The model under review builds one solid part; all positions refer to its coordinate system, in mm. Face numbers are marked on the shaded views. A direction names the side the tool comes from. Round coordinates to 2 decimals unless told otherwise and drop trailing zeros. Order: outer loops, then holes, each group sorted by start corner. A loop starts at its lowest first (then second) coordinate and runs counter-clockwise, first axis right, second up.
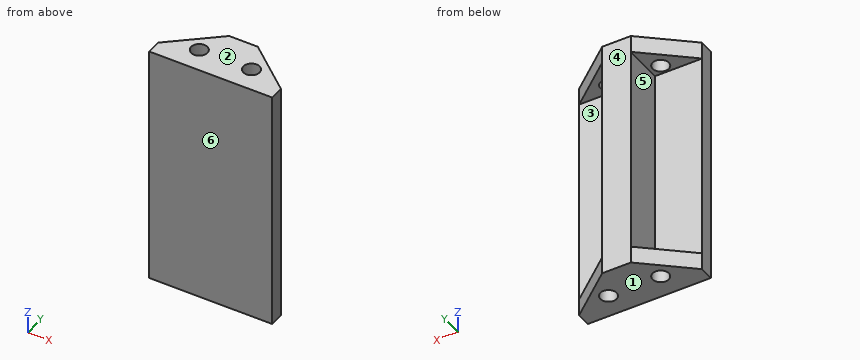
from build123d import *

# Parameters (mm, degrees)
SKETCH1_R           = 2.85
BOSS_EXTRUDE1_DEPTH = 85.7063165
CUT_EXTRUDE1_START  = -6
CUT_EXTRUDE1_DEPTH  = 73.706316
SKETCH3_R           = 2.85
CUT_EXTRUDE2_DEPTH  = 86.7063165


with BuildPart() as part:
    # Sketch1 → Boss-Extrude1 (new body)
    with BuildSketch(Plane.XY):
        Polygon((-21.5, -9.422571957), (21.5, -9.422571957), (21.5, -4.422571957), (5, 9.422571957), (-5, 9.422571957), (-21.5, -4.422571957), align=None)
        with Locations((-9.125, -0.961285979)):
            Circle(SKETCH1_R, mode=Mode.SUBTRACT)
        with Locations((9.125, -0.961285979)):
            Circle(SKETCH1_R, mode=Mode.SUBTRACT)
        with Locations((-9.125, -0.961285979)):
            Circle(SKETCH1_R)
        with Locations((9.125, -0.961285979)):
            Circle(SKETCH1_R)
    extrude(amount=BOSS_EXTRUDE1_DEPTH)

    # Sketch2 → Cut-Extrude1 (cut)
    with BuildSketch(Plane(origin=(0, 0, 0), x_dir=(-1, 0, 0), z_dir=(0, 0, -1)).offset(CUT_EXTRUDE1_START)):
        Polygon((5, 9.422571957), (21.5, -4.422571957), (5, -4.422571957), align=None)
        Polygon((-21.5, -4.422571957), (-5, 9.422571957), (-5, -4.422571957), align=None)
    extrude(amount=-CUT_EXTRUDE1_DEPTH, mode=Mode.SUBTRACT)

    # Sketch3 → Cut-Extrude2 (cut, through all)
    with BuildSketch(Plane(origin=(0, 0, 0), x_dir=(-1, 0, 0), z_dir=(0, 0, -1))):
        with Locations((9.125, -0.961285979)):
            Circle(SKETCH3_R)
        with Locations((-9.125, -0.961285979)):
            Circle(SKETCH3_R)
    extrude(amount=-CUT_EXTRUDE2_DEPTH, mode=Mode.SUBTRACT)


solid = part.part
(1) The part is to be moulded in two halves that separate along Z. For the marked faces 1, 2, 3 and 4, say which applies: pulls with the +Z half, pulls with the -Z half, needs draft (parallel to the pull), parting line crosses it, or undercut.
(2) We need section A-A (z = 55.5). Give the boundary of the cut face in (x, y).
(3) We need section B-B (y = -2.5). Give the boundary of the cut face in (x, z).
(4) We need section C-C (x = -11). Give the boundary of the cut face in (y, z), and give its area (3 significant figures).
(5) To check wall thickness, follow L1, parallel to Z at x = 12, y = 2.25; L2, parallel to X at y = 2.5, z = 68; L3, parallel to Y at x = -9, z = 65.5. State the ranges of each line that lie inside material, in increasing order.
(6) Clearance check with flat-ended pins moving along their axes: P1, Ø1.5, axis at y = -1, z = 75.5, coming from the +X side; P2, Ø5, axis at x = -16, z = 42, coming from the +Y side; P3, Ø5, axis at x = 9.12, y = -0.96, coming from the -Z side; P4, Ø7, axis at x = -15.5, y = 2, coming from the -Z side. State where each tip first meets the part, or that it passes through.
(7) Tool access review of the marked faces 5 and 6: name each direction out of +Z, -Z, +X, -X, +Y, -Y from which nothing blocks a thin tool from reaching the whole face with its end or side.
(8) We need section D-D (y = 3.25). Give the boundary of the cut face in (x, z), and give its area (3 significant figures).
Verdict:
1. face 1: pulls with the -Z half
1. face 2: pulls with the +Z half
1. face 3: undercut
1. face 4: needs draft
2. outline: (-21.5, -9.42) - (21.5, -9.42) - (21.5, -4.42) - (5, -4.42) - (5, 9.42) - (-5, 9.42) - (-5, -4.42) - (-21.5, -4.42) - close
3. outline: (-19.21, 0) - (-11.52, 0) - (-11.52, 6) - (-19.21, 6) - close; (-19.21, 79.71) - (-11.52, 79.71) - (-11.52, 85.71) - (-19.21, 85.71) - close; (-6.73, 0) - (6.73, 0) - (6.73, 6) - (5, 6) - (5, 79.71) - (6.73, 79.71) - (6.73, 85.71) - (-6.73, 85.71) - (-6.73, 79.71) - (-5, 79.71) - (-5, 6) - (-6.73, 6) - close; (11.52, 0) - (19.21, 0) - (19.21, 6) - (11.52, 6) - close; (11.52, 79.71) - (19.21, 79.71) - (19.21, 85.71) - (11.52, 85.71) - close
4. outline: (-9.42, 0) - (-3.11, 0) - (-3.11, 6) - (-4.42, 6) - (-4.42, 79.71) - (-3.11, 79.71) - (-3.11, 85.71) - (-9.42, 85.71) - close; (1.19, 0) - (4.39, 0) - (4.39, 6) - (1.19, 6) - close; (1.19, 79.71) - (4.39, 79.71) - (4.39, 85.71) - (1.19, 85.71) - close
4. area: 483 mm2
5. L1: z = 0 to 6, 79.71 to 85.71
5. L2: x = -5 to 5
5. L3: y = -9.42 to -4.42
6. P1: stops at x = 5
6. P2: stops at y = -4.42
6. P3: passes through
6. P4: stops at z = 0
7. face 5: -X, +Y
7. face 6: +Z, -Z, +X, -X, -Y
8. outline: (-12.36, 0) - (12.36, 0) - (12.36, 6) - (5, 6) - (5, 79.71) - (12.36, 79.71) - (12.36, 85.71) - (-12.36, 85.71) - (-12.36, 79.71) - (-5, 79.71) - (-5, 6) - (-12.36, 6) - close
8. area: 1,030 mm2
